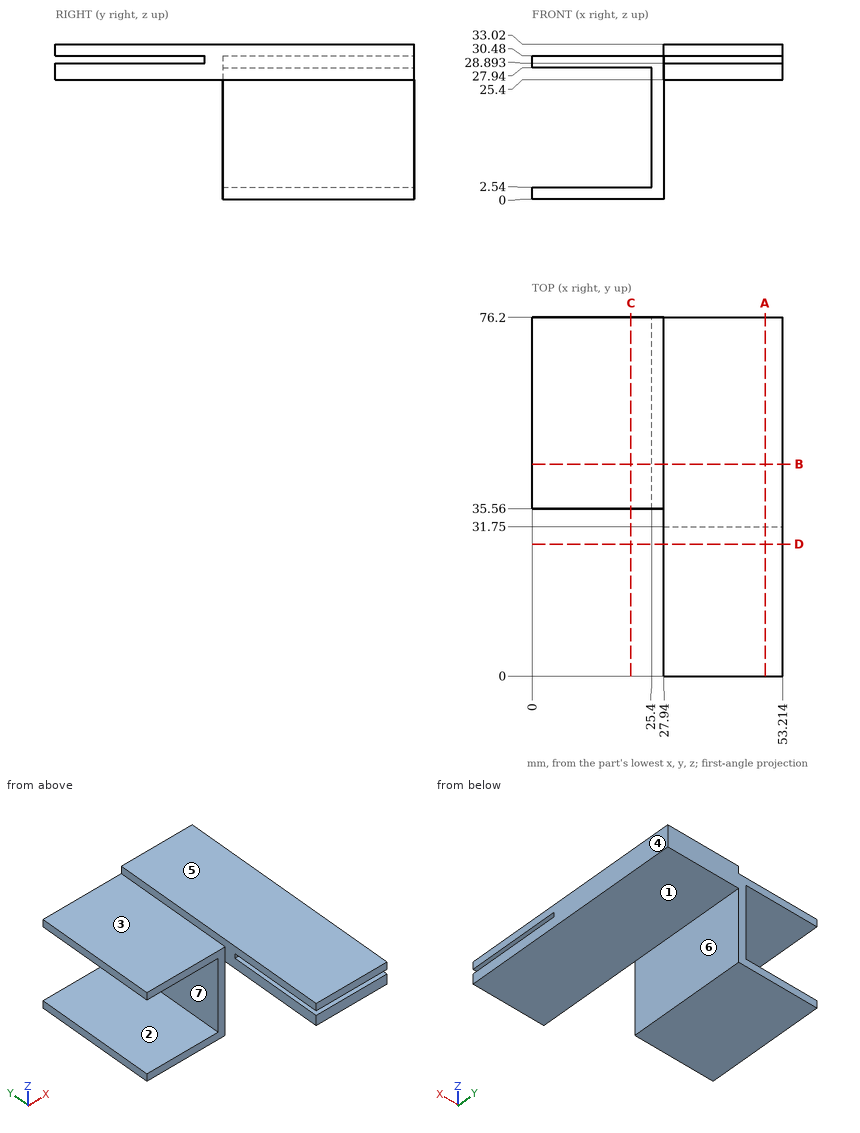
Design review of the part shown in the three views and the two pictorial views. Dimensions are in mm from the part's minimum x, y and z. A direction names the side the tool comes from. Give positions to 0.01 mm unless a question says otherwise; leave off trailing zeros. Loops run counter-clockwise (first coordinate to the right, second up) from the corner with the lowest first, then second, coordinate; pieces in that order, holes last. Notation, with made-up numbers: (69.5, -3) -> (75.5, -3) arc R25 ccw to (75.5, 17) -> close; hole circle Ø4 at (-39, 45.25). An arc over 180 degrees is marked (long way). One line per question, with ' | ' between items.
1) We need section A-A (x = 49.5). Write out the cut boundary in (y, z), plus the area to 3 significant figures.
Resolved:
outline: (0, 25.4) -> (76.2, 25.4) -> (76.2, 33.02) -> (0, 33.02) -> (0, 30.48) -> (31.75, 30.48) -> (31.75, 28.89) -> (0, 28.89) -> close | area: 530 mm2
2) We need section D-D (y = 28). Write out the cut boundary in (x, z) (1 decimal).
Resolved:
outline: (27.9, 25.4) -> (53.2, 25.4) -> (53.2, 28.9) -> (27.9, 28.9) -> close; (27.9, 30.5) -> (53.2, 30.5) -> (53.2, 33) -> (27.9, 33) -> close
3) The part is to be moulded in two halves that separate along Z. For the marked faces 1, 2, 3 and 4, say which applies: +Z half, -Z half, draft (parallel to the pull), parting line (faces both ways), or undercut.
Resolved:
face 1: -Z half | face 2: undercut | face 3: +Z half | face 4: draft
4) We need section C-C (x = 21). Write out the cut boundary in (y, z).
Resolved:
outline: (35.56, 0) -> (76.2, 0) -> (76.2, 2.54) -> (35.56, 2.54) -> close; (35.56, 27.94) -> (76.2, 27.94) -> (76.2, 30.48) -> (35.56, 30.48) -> close
5) For the marked faces 5, 6 and 7, list the 3-axis set-ups (+Z, -Z, +X, -X, +Y, -Y) from which the entire face can be reached by the end or side of a thin tool; tool diameter is ignored.
Resolved:
face 5: +Z, +X, -X, +Y, -Y | face 6: -Z, +X, +Y, -Y | face 7: -X, +Y, -Y
6) Insertion check: pin 1 Ø1.3 at (x, z) = (46.5, 29.5) entering from -Y; pin 2 Ø1.5 at (x, z) = (23.5, 6.5) entering from +Y; pin 3 Ø12.5 at (y, z) = (51, 14.5) entering from +X; pin 4 Ø1 at (y, z) = (65, 9.5) entering from -X. Each pin has a flat end and moves straight along its axis. Give the tip position at first contact, or say it passes through.
Resolved:
pin 1: stops at y = 0 | pin 2: passes through | pin 3: stops at x = 27.94 | pin 4: stops at x = 25.4
7) We need section B-B (y = 45). Write out the cut boundary in (x, z) (1 decimal), plus the area to 3 significant figures.
Resolved:
outline: (0, 0) -> (27.9, 0) -> (27.9, 25.4) -> (53.2, 25.4) -> (53.2, 33) -> (27.9, 33) -> (27.9, 30.5) -> (0, 30.5) -> (0, 27.9) -> (25.4, 27.9) -> (25.4, 2.5) -> (0, 2.5) -> close | area: 399 mm2
8) To check wall thickness, follow probe 1 along Z at (x, y) = (5.5, 58); probe 2 along Z at (x, y) = (36.5, 19.5); probe 3 along X at (y, z) = (59, 10). State the ranges of each line that lie inside material, in increasing order.
Resolved:
probe 1: z = 0 to 2.54, 27.94 to 30.48 | probe 2: z = 25.4 to 28.89, 30.48 to 33.02 | probe 3: x = 25.4 to 27.94
